Design review of the part built by this model. Coordinates are the model's own, in mm. Coordinates: 2 decimals unless noted, no trailing zeros. Write each loop counter-clockwise with the first axis right and the second up, starting at its lowest first coordinate (ties: lowest second). Pieces come first, ordered by that corner, then holes. Notation, with made-up numbers: M 43.5,18 L 58.5,18 A20 ccw 58.5,27 Z; hole C -39,74.5 d5. An arc over 180 degrees is marked long. One line per question, with ' | ' between items.
from build123d import *

# Parameters (mm, degrees)
F1_DEPTH = 672
F3_DEPTH = 25


with BuildPart() as f1:
    # F0 (on Right) → F1 (new body)
    with BuildSketch(Plane.YZ):
        Polygon((-14, 0), (0, 0), (0, 40), (-11, 40), (-19, 25), (-19, 5), align=None)
    extrude(amount=F1_DEPTH)

    # F2 (on Front) → F3 (cut)
    with BuildSketch(Plane.XZ):
        Polygon((0, 40), (0, 0), (40, 40), align=None)
        Polygon((672, 40), (632, 40), (672, 0), align=None)
    extrude(amount=F3_DEPTH, mode=Mode.SUBTRACT)


solid = f1.part
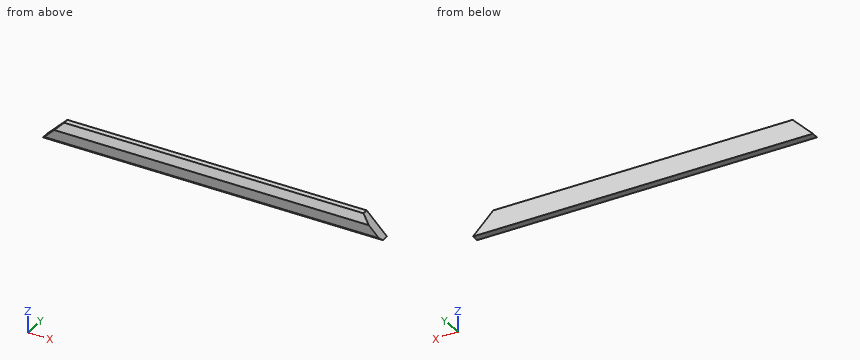
1. Take a section at A-A (x = 318). Write out the cut boundary in (y, z), then the cut area to 4 significant figures.
Answer sheet:
outline: M -19,5 L -14,0 L 0,0 L 0,40 L -11,40 L -19,25 Z | area: 687.5 mm^2
2. To check wall thickness, follow line 1 along Y through (x, z) = (564, 38); line 2 along X through (y, z) = (-4, 15); line 3 along X through (y, z) = (-13.5, 7). State the ranges of each line that lie inside material, in increasing order. Write a range as [from, to].
Answer sheet:
line 1: [-12.07, 0] | line 2: [15, 657] | line 3: [7, 665]
3. Take a section at B-B (z = 12). Write out the cut boundary in (x, y).
Answer sheet:
outline: M 12,-19 L 660,-19 L 660,0 L 12,0 Z
4. Take a section at C-C (y = -4.75). Write out the cut boundary in (x, z), then the cut area to 3 significant figures.
Answer sheet:
outline: M 0,0 L 672,0 L 632,40 L 40,40 Z | area: 25,300 mm^2
5. Insertion check: pin 1 Ø1.5 at (x, y) = (246.5, -15.5) entering from +Z; pin 2 Ø5 at (x, z) = (429, 28.5) entering from -Y; pin 3 Ø10 at (y, z) = (-13, 29) entering from +X. Each pin has a flat end and moves straight along its axis. Give the tip position at first contact, or say it passes through.
Answer sheet:
pin 1: z = 32.97 | pin 2: y = -18.47 | pin 3: x = 648
